Could you check a few things on this model? Use its own coordinates, in mm. A direction names the side the tool comes from. Give positions to 0.01 mm unless a question says otherwise; leave off trailing zeros. Order: outer loops, then holes, each group sorted by start corner. A loop starts at its lowest first (then second) coordinate and runs counter-clockwise, first axis right, second up.
from build123d import *

# Parameters (mm, degrees)
BOSS_EXTRU_7_DEPTH      = 30
ECHELLE1_SCALE          = 0.45
ESQUISSE2_W             = 105.662811699
ESQUISSE2_H             = 110
ENL_V_MAT_EXTRU_1_DEPTH = 22.7500001
ESQUISSE3_W             = 30
ESQUISSE3_H             = 6.75
ENL_V_MAT_EXTRU_3_DEPTH = 560.216594492


with BuildPart() as part:
    # Esquisse1 → Boss.-Extru.7 (new body)
    with BuildSketch(Plane(origin=(0, 0, 0), x_dir=(1, 0, 0), z_dir=(0, 1, 0))):
        with BuildLine():
            Line((130.068099718, -349.430080583), (176.932850794, 42.776117227))
            ThreePointArc((176.932850794, 42.776117227), (140.21219631, 65.055468432), (104.297030791, 41.49964449))
            ThreePointArc((104.297030791, 41.49964449), (83.352659725, 49.557480865), (63.285053961, 39.513248426))
            ThreePointArc((63.285053961, 39.513248426), (24.333712458, 39.346724586), (0.792917217, 8.313424819))
            add(Edge.make_bspline(
                [(0.792917217, 8.313424819), (-2.209813164, -2.681427076), (-5.40896856, -13.621959217)],
                knots=[0.221662646, 0.221662646, 0.221662646, 1, 1, 1], degree=2))
            ThreePointArc((-5.40896856, -13.621959217), (-34.929657478, -173.074330833), (-6.757332127, -332.770448419))
            add(Edge.make_bspline(
                [(-6.757332127, -332.770448419), (-2.007582254, -345.453681588), (0.57620201, -358.635638513)],
                knots=[0.963730152, 0.963730152, 0.963730152, 1.791334476, 1.791334476, 1.791334476], degree=2))
            ThreePointArc((0.57620201, -358.635638513), (69.060806185, -414.873028703), (129.997803695, -350.534335844))
            ThreePointArc((129.997803695, -350.534335844), (130.017666903, -349.981235195), (130.068099718, -349.430080583))
        make_face()
    extrude(amount=BOSS_EXTRU_7_DEPTH)


with BuildPart() as part_1:
    # Echelle1: scaled about (67.671552852, 15, 164.896156294)
    add(part.part.scale(ECHELLE1_SCALE).moved(Location((37.219354069, 8.25, 90.692885962))))

    # Esquisse2 → Enlèv. mat.-Extru.1 (cut, through all)
    with BuildSketch(Plane(origin=(0, 0, 0), x_dir=(1, 0, 0), z_dir=(0, 1, 0))):
        with Locations((71.147737752, -83.392019497)):
            Rectangle(ESQUISSE2_W, ESQUISSE2_H)
    extrude(amount=ENL_V_MAT_EXTRU_1_DEPTH, mode=Mode.SUBTRACT)

    # Esquisse3 → Enlèv. mat.-Extru.3 (cut, through all)
    with BuildSketch(Plane(origin=(580.715772067, 0, 0), x_dir=(0, 0, -1), z_dir=(1, 0, 0))):
        with Locations((-153.392019497, 18.375)):
            Rectangle(ESQUISSE3_W, ESQUISSE3_H)
    extrude(amount=-ENL_V_MAT_EXTRU_3_DEPTH, mode=Mode.SUBTRACT)


solid = part_1.part
Item 1: Please list where these lines run through material, in increasing order: line 1 along Y through (x, z) = (30, 161.5); line 2 along X through (y, z) = (13.75, 221); line 3 along X through (y, z) = (19.25, 169.5).
Findings:
line 1: y = 8.25 to 15
line 2: x = 28.08 to 98.97
line 3: x = 21.5 to 105.12
Item 2: For pin 1 (6 mm diameter, centred on y = 15.5, z = 234.5, fed in from -X); pin 2 (4 mm diameter, centred on y = 18.5, z = 252.5, fed in from +X); pin 3 (1 mm diameter, centred on y = 13, z = 248, fed in from +X), each with a flat end and sliding along its axis, tell me the tip position at first contact or that it passes through.
Findings:
pin 1: stops at x = 31.11
pin 2: stops at x = 95.63
pin 3: stops at x = 95.8
Item 3: Imagine slicing it at B-B on z = 149. List the corners of the cut face in (x, y) for me.
Findings:
outline: (22.52, 8.25) - (107.57, 8.25) - (107.57, 15) - (22.52, 15) - close
Item 4: Imagine slicing it at A-A on x = 46.5. List the corners of the cut face in (y, z) for me, then the cut area to 3 significant figures.
Findings:
outline: (8.25, 138.39) - (15, 138.39) - (15, 168.39) - (21.75, 168.39) - (21.75, 269.57) - (8.25, 269.57) - close
area: 1,570 mm2
Item 5: Imagine slicing it at D-D on z = 216. List the corners of the cut face in (x, y) for me.
Findings:
outline: (26.85, 8.25) - (99.57, 8.25) - (99.57, 21.75) - (26.85, 21.75) - close
Item 6: Imagine slicing it at C-C on x = 71. List the corners of the cut face in (y, z) for me, then the cut area to 3 significant figures.
Findings:
outline: (8.25, 138.39) - (15, 138.39) - (15, 168.39) - (21.75, 168.39) - (21.75, 277.09) - (8.25, 277.09) - close
area: 1,670 mm2
Item 7: For faces 1 (the flat face through (64, 18, 168.392)), 2 (the flat face through (66, 12, 138.392)), which set-ups out of +Z, -Z, +X, -X, +Y, -Y let a thin tool reach every point of the face, with its end or its side?
Findings:
face 1: -Z, +X, -X, +Y
face 2: -Z, +X, -X, +Y, -Y
